Build history of the part. All positions in model axes, mm. Face numbers are marked on the shaded views. A direction names the side the tool comes from. Give positions to 0.01 mm unless a question says otherwise; leave off trailing zeros. Order: outer loops, then holes, each group sorted by start corner. A loop starts at its lowest first (then second) coordinate and runs counter-clockwise, first axis right, second up. Notation, with made-up numbers: (88, 9.5) -> (107, 9.5) arc R17 cw to (107, 22.5) -> close; hole circle Ø6 at (9.5, 83). An arc over 180 degrees is marked (long way). One line per item, written item: value. Start each with the question number.
(1) Saw through at A-A on z = 0. Give the cut face in (x, y) (3 decimals).
(2) Two-plate mould, pull along X, no slides. Class the marked faces 1, 2, 3 and 4: +X half, -X half, draft (parallel to the pull), parting line (faces both ways), or undercut.
(3) Saw through at B-B on y = 3.5. Give the cut face in (x, z) (3 decimals), plus the area to 3 significant figures.
(4) Saw through at D-D on y = 8.75. Give the cut face in (x, z) (3 decimals), plus the area to 3 significant figures.
(5) Saw through at C-C on x = 0. Give the cut face in (y, z) (3 decimals), plus the area to 3 significant figures.
(6) Probe line 1 (X direction, y = 3.5, z = 0) (3 decimals); line 2 (Z direction, x = -7.5, y = 3.5) (3 decimals); line 3 (X direction, y = 2.75, z = 0) (3 decimals). List the from-to ranges inside material, lowest first.
(7) Which spindle directions (+Z, -Z, +X, -X, +Y, -Y) get a long thin tool onto all of the face, cutting with end or side? Do the marked faces 5, 6 and 7. Say none if no direction does.
(8) Pin check, flat tips, straight feed: pin 1 (2 mm diameter, centred on x = -4, y = 7.5, fed in from -Z); pin 2 (1.3 mm diameter, centred on x = 4, y = 9, fed in from -Z); pin 3 (4 mm diameter, centred on y = 2.5, z = -3.5, fed in from +X); pin 4 (5 mm diameter, centred on x = 0, z = 0, fed in from -Y). Stop position of each tip, or through.
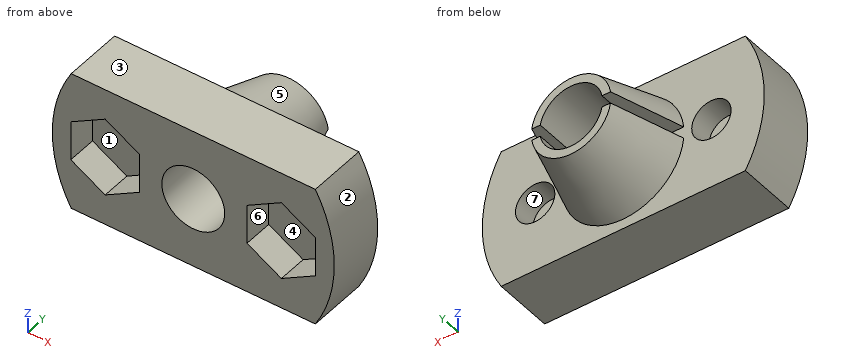
```python
from build123d import *

# Parameters (mm, degrees)
SKETCH1_R           = 12
SKETCH1_R_2         = 2.675
BOSS_EXTRUDE1_DEPTH = 5
SKETCH2_R           = 5.16665
SKETCH2_R_2         = 2.675
BOSS_EXTRUDE2_DEPTH = 6
CHAMFER1_SIZE       = 6
CHAMFER1_SIZE_2     = 1.77728097
SKETCH3_R           = 1.675
CUT_EXTRUDE1_DEPTH  = 6
CUT_EXTRUDE2_DEPTH  = 2.5
SKETCH5_W           = 10.3333
SKETCH5_H           = 1
CUT_EXTRUDE3_DEPTH  = 6
CUT_EXTRUDE4_DEPTH  = 10
BOSS_EXTRUDE3_START = -0.5
SKETCH7_R           = 1.706123363
SKETCH7_R_2         = 1.675
BOSS_EXTRUDE3_DEPTH = 0.5


with BuildPart() as part:
    # Sketch1 → Boss-Extrude1 (new body)
    with BuildSketch(Plane(origin=(0, 0, 0), x_dir=(1, 0, 0), z_dir=(0, 1, 0))):
        with Locations(Location((0, 0, 0), (0, 0, 270))):
            Circle(SKETCH1_R)
        with Locations(Location((0, 0, 0), (0, 0, 270))):
            Circle(SKETCH1_R_2, mode=Mode.SUBTRACT)
    extrude(amount=BOSS_EXTRUDE1_DEPTH)

    # Sketch2 → Boss-Extrude2 (add)
    with BuildSketch(Plane(origin=(0, 5, 0), x_dir=(1, 0, 0), z_dir=(0, 1, 0))):
        with Locations(Location((0, 0, 0), (0, 0, 270))):
            Circle(SKETCH2_R)
        with Locations(Location((0, 0, 0), (0, 0, 270))):
            Circle(SKETCH2_R_2, mode=Mode.SUBTRACT)
    extrude(amount=BOSS_EXTRUDE2_DEPTH)

    # Chamfer1
    # the kernel refuses this chamfer: 6, 1.77728097 mm, written as the material it takes off along each edge
    with BuildSketch(Plane(origin=(0, 11, 0), x_dir=(0, 0, 1), z_dir=(-1, 0, 0))) as chamfer1_piece_1_section:
        Polygon((5.16665, -CHAMFER1_SIZE), (5.16665 - CHAMFER1_SIZE_2, 0), (5.16665, 0), align=None)
    chamfer1_piece_1 = revolve(axis=Axis((0, 11, 0), (0, 1, 0)), mode=Mode.PRIVATE)
    chamfer1_piece_1 = split(chamfer1_piece_1, bisect_by=Plane(origin=(0, 5, -4.298679157), z_dir=(0, 1, 0)), keep=Keep.TOP, mode=Mode.PRIVATE)
    add(chamfer1_piece_1, mode=Mode.SUBTRACT)

    # Sketch3 → Cut-Extrude1 (cut)
    with BuildSketch(Plane(origin=(0, 5, 0), x_dir=(1, 0, 0), z_dir=(0, 1, 0))):
        with Locations(Location((-7.5, 0, 0), (0, 0, 270))):
            Circle(SKETCH3_R)
        with Locations(Location((7.5, 0, 0), (0, 0, 270))):
            Circle(SKETCH3_R)
    extrude(amount=-CUT_EXTRUDE1_DEPTH, mode=Mode.SUBTRACT)

    # Sketch4 → Cut-Extrude2 (cut)
    with BuildSketch(Plane.XZ):
        Polygon((-10.425, -1.688749537), (-7.5, -3.377499075), (-4.575, -1.688749537), (-4.575, 1.688749537), (-7.5, 3.377499075), (-10.425, 1.688749537), align=None)
        Polygon((10.425, 1.688749537), (10.425, -1.688749537), (7.5, -3.377499075), (4.575, -1.688749537), (4.575, 1.688749537), (7.5, 3.377499075), align=None)
    extrude(amount=-CUT_EXTRUDE2_DEPTH, mode=Mode.SUBTRACT)

    # Sketch5 → Cut-Extrude3 (cut)
    with BuildSketch(Plane(origin=(0, 5, 0), x_dir=(1, 0, 0), z_dir=(0, 1, 0))):
        Rectangle(SKETCH5_W, SKETCH5_H)
    extrude(amount=CUT_EXTRUDE3_DEPTH, mode=Mode.SUBTRACT)

    # Sketch6 → Cut-Extrude4 (cut)
    with BuildSketch(Plane.XZ):
        with BuildLine():
            Line((-10.392304845, 6), (10.392304845, 6))
            ThreePointArc((10.392304845, 6), (0, 12), (-10.392304845, 6))
        make_face()
        with BuildLine():
            Line((-10.392304845, -6), (10.392304845, -6))
            ThreePointArc((10.392304845, -6), (0, -12), (-10.392304845, -6))
        make_face()
    extrude(amount=-CUT_EXTRUDE4_DEPTH, mode=Mode.SUBTRACT)

    # Sketch7 → Boss-Extrude3 (add)
    with BuildSketch(Plane.XZ.offset(-2.5).offset(BOSS_EXTRUDE3_START)):
        with Locations((7.5, 0)):
            Circle(SKETCH7_R)
        with Locations(Location((-7.5, 0, 0), (0, 0, 90))):
            Circle(SKETCH7_R_2)
    extrude(amount=BOSS_EXTRUDE3_DEPTH)


solid = part.part
```
Results below:
1. outline: (-12, 0) -> (-10.425, 0) -> (-10.425, 2.5) -> (-4.575, 2.5) -> (-4.575, 0) -> (-2.675, 0) -> (-2.675, 5) -> (-5.825, 5) -> (-5.825, 3) -> (-9.175, 3) -> (-9.175, 5) -> (-12, 5) -> close; (2.675, 0) -> (4.575, 0) -> (4.575, 2.5) -> (10.425, 2.5) -> (10.425, 0) -> (12, 0) -> (12, 5) -> (9.175, 5) -> (9.175, 3) -> (5.825, 3) -> (5.825, 5) -> (2.675, 5) -> close
2. face 1: undercut
2. face 2: +X half
2. face 3: draft
2. face 4: undercut
3. outline: (-10.392, -6) -> (10.392, -6) arc R12 ccw to (10.392, 6) -> (-10.392, 6) arc R12 ccw to start; hole circle Ø3.35 at (-7.5, 0); hole circle Ø5.35 at (0, 0); hole circle Ø3.35 at (7.5, 0)
3. area: 235 mm²
4. outline: (-4.025, -0.5) arc R4.056 ccw to (4.025, -0.5) -> (2.628, -0.5) arc R2.675 cw to (-2.628, -0.5) -> close; (-4.025, 0.5) -> (-2.628, 0.5) arc R2.675 cw to (2.628, 0.5) -> (4.025, 0.5) arc R4.056 ccw to start
4. area: 26.4 mm²
5. outline: (0, -6) -> (5, -6) -> (5, -5.167) -> (11, -3.389) -> (11, -2.675) -> (0, -2.675) -> close; (0, 2.675) -> (11, 2.675) -> (11, 3.389) -> (5, 5.167) -> (5, 6) -> (0, 6) -> close
5. area: 52.5 mm²
6. line 1: x = -12 to -9.175, -5.825 to -2.675, 2.675 to 5.825, 9.175 to 12
6. line 2: z = -6 to -1.675, 1.675 to 6
6. line 3: x = -12 to -2.675, 2.675 to 12
7. face 5: +Z, +Y
7. face 6: -Y
7. face 7: +Y
8. pin 1: stops at z = -3.34
8. pin 2: stops at z = -2.21
8. pin 3: stops at x = 11.91
8. pin 4: passes through
